```python
from build123d import *

# Parameters (mm, degrees)
BOSS_EXTRUDE1_DEPTH             = 3.175
CUT_EXTRUDE1_DEPTH              = 165.102970266
FILLET4_R                       = 3.175
FILLET5_R                       = 3.175
FILLET6_R                       = 3.175
FILLET7_R                       = 1.27
F_2_56_TAPPED_HOLE1_D           = 1.778
F_2_56_TAPPED_HOLE1_ON_FACE_2_D = 1.778


with BuildPart() as part:
    # Sketch1 → Boss-Extrude1 (new body)
    with BuildSketch(Plane(origin=(0, 0, 0), x_dir=(0, 0, -1), z_dir=(1, 0, 0))):
        with BuildLine():
            Line((0, 0), (142.24, 0))
            Line((142.24, 0), (142.24, 3.175))
            Line((142.24, 3.175), (148.59, 3.175))
            Line((148.59, 3.175), (154.94, 44.45))
            Line((154.94, 44.45), (148.59, 44.45))
            Line((148.59, 44.45), (148.59, 47.625))
            Line((148.59, 47.625), (154.94, 47.625))
            Line((154.94, 47.625), (154.94, 53.975))
            Line((154.94, 53.975), (142.24, 53.975))
            Line((142.24, 53.975), (0, 9.113473275))
            ThreePointArc((0, 9.113473275), (-3.148798139, 6.856769541), (-4.353876774, 3.175))
            Line((-4.353876774, 3.175), (0, 3.175))
            Line((0, 3.175), (0, 0))
        make_face()
    extrude(amount=BOSS_EXTRUDE1_DEPTH)

    # Sketch2 → Cut-Extrude1 (cut, through all)
    with BuildSketch(Plane(origin=(3.175, 0, 0), x_dir=(0, 0, -1), z_dir=(1, 0, 0))):
        Polygon((142.24, 51.311663913), (142.24, 6.450137188), (111.020554533, 6.450137188), (119.363152794, 44.096462195), align=None)
        Polygon((108.873959331, 40.788242054), (101.264477824, 6.450137188), (70.045032356, 6.450137188), (75.30854025, 30.201937603), align=None)
        Polygon((71.812142429, 29.099197556), (66.793006787, 6.450137188), (35.573561319, 6.450137188), (38.246723348, 18.512893105), align=None)
        Polygon((0, 6.450137188), (34.750325527, 17.410153058), (32.32153575, 6.450137188), align=None)
    extrude(amount=-CUT_EXTRUDE1_DEPTH, mode=Mode.SUBTRACT)

    # Fillet4
    fillet4_edges = [part.edges().sort_by_distance(p)[0] for p in [
        (1.5875, 44.096462195, -119.363152794),
        (1.5875, 6.450137188, -142.24),
        (1.5875, 6.450137188, -111.020554533),
        (1.5875, 6.450137188, -32.32153575),
        (1.5875, 18.512893105, -38.246723348),
        (1.5875, 6.450137188, -66.793006787),
        (1.5875, 6.450137188, -35.573561319),
        (1.5875, 30.201937603, -75.30854025),
        (1.5875, 6.450137188, -101.264477824),
        (1.5875, 6.450137188, -70.045032356),
    ]]
    fillet(fillet4_edges, radius=FILLET4_R)

    # Fillet5
    fillet5_edges = [part.edges().sort_by_distance(p)[0] for p in [
        (1.5875, 51.311663913, -142.24),
        (1.5875, 17.410153058, -34.750325527),
        (1.5875, 29.099197556, -71.812142429),
        (1.5875, 40.788242054, -108.873959331),
    ]]
    fillet(fillet5_edges, radius=FILLET5_R)

    # Fillet6
    fillet6_edges = [part.edges().sort_by_distance(p)[0] for p in [
        (1.5875, 53.975, -154.94),
    ]]
    fillet(fillet6_edges, radius=FILLET6_R)

    # Fillet7
    fillet7_edges = [part.edges().sort_by_distance(p)[0] for p in [
        (1.5875, 6.450137188, 0),
    ]]
    fillet(fillet7_edges, radius=FILLET7_R)

    # 2-56 Tapped Hole1 (through all)
    with Locations(Plane(origin=(3.175, 35.052107057, -112.480843865), x_dir=(0, 0, 1), z_dir=(1, 0, 0))):
        with Locations((0, 0), (2.747718528, 12.399195251), (4.121577793, 18.598792877)):
            Hole(F_2_56_TAPPED_HOLE1_D / 2)

    # 2-56 Tapped Hole1 on face 2 (through all)
    with Locations(Plane(origin=(524.251745337, 38.733811309, 0), x_dir=(0, 0, 1), z_dir=(1, 0, 0))):
        with Locations((0, 0)):
            Hole(F_2_56_TAPPED_HOLE1_ON_FACE_2_D / 2)


solid = part.part
```
Source: CAD feature listing. Evaluate the final solid. Frame: model axes, mm. A direction names the side the tool comes from. Round coordinates to 2 decimals unless told otherwise and drop trailing zeros. Loops run counter-clockwise (first coordinate to the right, second up) from the corner with the lowest first, then second, coordinate; pieces in that order, holes last. Notation, with made-up numbers: M 38,8 L 79,8 A19 ccw 79,34 Z; hole C -36,43.5 d9. An arc over 180 degrees is marked long. Use a Markdown table: item, result. Add a question column.
1. Pull-direction query (Y, two-part tool) for faces 5 (the flat face through (0, 17, -104)), 6 (the flat face through (2, 0, -70)), 7 (the flat face through (1.61, 47.29, -129.49)); classes: +Y half, -Y half, draft (parallel to the pull), parting line (faces both ways), or undercut.
2. Ray query, line 1 along Y through (x, z) = (0.25, -109); line 2 along Z through (x, y) = (1.55, 3); line 3 along Y through (x, z) = (1.2, -124). Return the intervals inside material, ascending. Write a range as [from, to].
3. Cut plane A-A, the plane z = -132.5. Output: boundary loops of the cut face in (x, y) (3 decimals), and give its area (3 significant figures).
4. Cut plane D-D, the plane y = 5. Output: boundary loops of the cut face in (x, z) (3 decimals), and give its area (3 significant figures).
5. Set-up query: faces 1 (the flat face through (2, 49, -154.94)), 2 (the flat face through (2, 2, -142.24)), 3 (the flat face through (2, 6.45, -127)), 4 (the flat face through (2, 47.625, -152)). Return all of +Z, -Z, +X, -X, +Y, -Y with unobstructed straight access to the full face (end or side cutting, diameter ignored); none if empty.
6. Contact query for flat-ended pins moving along their axis: pin 1 (1.6 mm diameter, centred on x = 2, z = -17.5, fed in from +Y); pin 2 (1.6 mm diameter, centred on x = 2, y = 1.5, fed in from -Z). Output: stop coordinate, or through.
7. Cut plane B-B, the plane y = 14. Output: boundary loops of the cut face in (x, z) (3 decimals).
8. Cut plane C-C, the plane x = 0.75. State how many separate pieces and enclosed holes the cut face has, and give its area (3 significant figures).
Solution:
| question | item | result |
|---|---|---|
| 1 | face 5 | draft |
| 1 | face 6 | -Y half |
| 1 | face 7 | undercut |
| 2 | line 1 | y = [0, 15.84], [17.07, 22.15], [23.16, 43.49] |
| 2 | line 2 | z = [-142.24, 0] |
| 2 | line 3 | y = [0, 6.45], [45.56, 48.22] |
| 3 | outline | M 0,0 L 3.175,0 L 3.175,6.45 L 0,6.45 Z; M 0,48.24 L 3.175,48.24 L 3.175,50.903 L 0,50.903 Z |
| 3 | area | 28.9 mm2 |
| 4 | outline | M 0,-148.871 L 3.175,-148.871 L 3.175,4.08 L 0,4.08 Z |
| 4 | area | 486 mm2 |
| 5 | face 1 | -Z, +X, -X, +Y, -Y |
| 5 | face 2 | -Z, +X, -X, -Y |
| 5 | face 3 | +X, -X |
| 5 | face 4 | -Z, +X, -X |
| 6 | pin 1 | stops at y = 14.89 |
| 6 | pin 2 | stops at z = -142.24 |
| 7 | outline | M 0,-150.255 L 3.175,-150.255 L 3.175,-142.24 L 0,-142.24 Z; M 0,-112.694 L 3.175,-112.694 L 3.175,-102.938 L 0,-102.938 Z; M 0,-71.718 L 3.175,-71.718 L 3.175,-68.466 L 0,-68.466 Z; M 0,-37.247 L 3.175,-37.247 L 3.175,-33.37 L 0,-33.37 Z; M 0,-23.938 L 3.175,-23.938 L 3.175,-15.493 L 0,-15.493 Z |
| 8 | separate pieces | 1 |
| 8 | enclosed holes | 7 |
| 8 | area | 2,320 mm2 |
